Here's how the part is built. I have some questions about the finished solid (model axes, mm). A direction names the side the tool comes from. Give positions to 0.01 mm unless a question says otherwise; leave off trailing zeros. Order: outer loops, then holes, each group sorted by start corner. A loop starts at its lowest first (then second) coordinate and runs counter-clockwise, first axis right, second up. Notation, with made-up numbers: M -36,-7 L -9,-7 A37 cw -9,29 Z; hole C -11.75,52 d6. An arc over 180 degrees is marked long. Use one line per item in the form item = value.
from build123d import *

# Parameters (mm, degrees)
BASE_EXTRUSION_DEPTH    = 2
ESQUISSE2_R             = 2.5
ENL_V_MAT_EXTRU_1_DEPTH = 2


with BuildPart() as part:
    # Esquisse1 → Base-Extrusion (new body)
    with BuildSketch(Plane.XY):
        with BuildLine():
            Line((0, 0), (6, 0))
            Line((6, 0), (6, 4.583801513))
            ThreePointArc((6, 4.583801513), (3, 20), (0, 4.583801513))
            Line((0, 4.583801513), (0, 0))
        make_face()
    extrude(amount=-BASE_EXTRUSION_DEPTH)

    # Esquisse2 → Enlèv. mat.-Extru.1 (cut)
    with BuildSketch(Plane.XY):
        with Locations((3, 12)):
            Circle(ESQUISSE2_R)
    extrude(amount=-ENL_V_MAT_EXTRU_1_DEPTH, mode=Mode.SUBTRACT)


solid = part.part
Q1. I want a section at B-B on y = 12. Write out the boundary of the cut face in (x, z).
Found:
outline = M -5,-2 L 0.5,-2 L 0.5,0 L -5,0 Z; M 5.5,-2 L 11,-2 L 11,0 L 5.5,0 Z
Q2. I'm going to push flat-ended pins straight in: pin 1 Ø0.6 at (y, z) = (2.5, -1.5) entering from +X; pin 2 Ø3 at (x, y) = (-1.5, 10.5) entering from +Z. Where does each tip first touch, or does it pass through?
Found:
pin_1 = 6
pin_2 = 0
Q3. I want a section at C-C on z = -0.55. Write out the boundary of the cut face in (x, y).
Found:
outline = M 0,0 L 6,0 L 6,4.58 A8 ccw long 0,4.58 Z; hole C 3,12 d5
Q4. I need wall thicknesses on L1, parallel to Y at x = 3.25, z = -1.5; L2, parallel to Y at x = 2.25, z = -0.8; L3, parallel to Y at x = 9, z = -0.5. Which ranges of each line are inside material? Lowest first, please.
Found:
L1 = 0 to 9.51, 14.49 to 20
L2 = 0 to 9.62, 14.38 to 19.96
L3 = 6.71 to 17.29
Q5. I want a section at D-D on y = 5.75. Write out the boundary of the cut face in (x, z).
Found:
outline = M -1.99,-2 L 7.99,-2 L 7.99,0 L -1.99,0 Z
Q6. I want a section at A-A on x = 3. Write out the boundary of the cut face in (y, z), then the cut area to 3 significant figures.
Found:
outline = M 0,-2 L 9.5,-2 L 9.5,0 L 0,0 Z; M 14.5,-2 L 20,-2 L 20,0 L 14.5,0 Z
area = 30.0 mm²
Q7. Thinking about a two-plate mould opening in Z: for faces 1 (the face through (1, 10, -2)), 2 (the face through (1, 10, 0)), 3 (the face through (3, 0, -1)), which applies, +Z half, -Z half, draft (parallel to the pull), parting line (faces both ways), or undercut?
Found:
face_1 = -Z half
face_2 = +Z half
face_3 = draft
Q8. On a 3-axis mill with a long thin cutter (end or side, diameter ignored), from which of +Z, -Z, +X, -X, +Y, -Y can I reach the whole of each face in a straight line? I mean faces 4 (the face through (2.46, 9.56, -0.99)), 5 (the face through (6, 2, -1)), 6 (the face through (0, 2, -1)). Say none if no direction works.
Found:
face_4 = +Z, -Z
face_5 = +Z, -Z, +X, -Y
face_6 = +Z, -Z, -X, -Y
